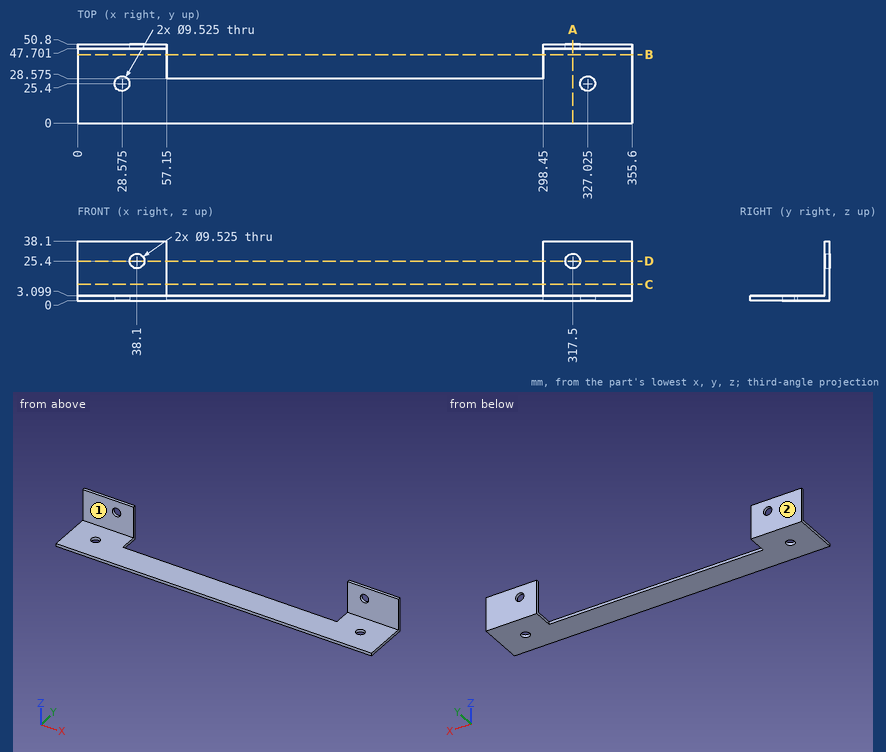
The figure shows three views and two pictorial views of one solid part (mm, origin at its lowest corner). Answer the questions. A direction names the side the tool comes from. Give positions to 0.01 mm unless a question says otherwise; leave off trailing zeros. Loops run counter-clockwise (first coordinate to the right, second up) from the corner with the lowest first, then second, coordinate; pieces in that order, holes last. Notation, with made-up numbers: (87, 87) -> (118, 87) arc R22 ccw to (118, 125) -> close; hole circle Ø8 at (39.5, 14.25). An arc over 180 degrees is marked (long way). Put each result on its own line as item: value. Start each with the question number.
Item 1: The part is cut by section C-C (z = 10.5). Give the vertices of the cut face in (x, y).
Item 2: The part is cut by section B-B (y = 44). Give the vertices of the cut face in (x, z), then the cut area to 3 significant figures.
Item 3: Each of these flat-tipped pins is pushed along its axis until it touches: P1, Ø4, axis at x = 138, y = 23, coming from the +Z side; P2, Ø3.5, axis at x = 162.5, z = 1, coming from the +Y side (3 decimals); P3, Ø10, axis at x = 317.5, z = 19.5, coming from the -Y side. Where does it stop, or does it pass through?
Item 4: The part is cut by section A-A (x = 317.5). Give the vertices of the cut face in (y, z), then the cut area to 3 significant figures.
Item 5: Which of the six approach directions +Z, -Z, +X, -X, +Y, -Y give full straight-line access (tool end or side, diameter ignored) to the marked faces 1 and 2?
Item 6: Find the intervals of material crossed by L1, parallel to X at y = 48, z = 25; L2, parallel to Z at x = 38.1, y = 49.8; L3, parallel to Y at x = 203, z = 3 (3 decimals), in increasing order. Write a range as [from, to].
Item 7: The part is cut by section D-D (z = 25.4). Give the vertices of the cut face in (x, y).
Answers below:
1. outline: (0, 47.7) -> (57.15, 47.7) -> (57.15, 50.8) -> (0, 50.8) -> close; (298.45, 47.7) -> (355.6, 47.7) -> (355.6, 50.8) -> (298.45, 50.8) -> close
2. outline: (0, 0) -> (57.15, 0) -> (57.15, 3.1) -> (0, 3.1) -> close; (298.45, 0) -> (355.6, 0) -> (355.6, 3.1) -> (298.45, 3.1) -> close
2. area: 354 mm2
3. P1: z = 3.1
3. P2: y = 28.575
3. P3: y = 47.7
4. outline: (0, 0) -> (50.8, 0) -> (50.8, 20.64) -> (47.7, 20.64) -> (47.7, 3.1) -> (0, 3.1) -> close; (47.7, 30.16) -> (50.8, 30.16) -> (50.8, 38.1) -> (47.7, 38.1) -> close
4. area: 236 mm2
5. face 1: +Z, +X, -X, -Y
5. face 2: +Z, -Z, +X, -X, +Y
6. L1: [0, 33.35], [42.85, 57.15], [298.45, 312.75], [322.25, 355.6]
6. L2: [0, 20.64], [30.16, 38.1]
6. L3: [0, 28.575]
7. outline: (0, 47.7) -> (33.34, 47.7) -> (33.34, 50.8) -> (0, 50.8) -> close; (42.86, 47.7) -> (57.15, 47.7) -> (57.15, 50.8) -> (42.86, 50.8) -> close; (298.45, 47.7) -> (312.74, 47.7) -> (312.74, 50.8) -> (298.45, 50.8) -> close; (322.26, 47.7) -> (355.6, 47.7) -> (355.6, 50.8) -> (322.26, 50.8) -> close
